```python
from build123d import *

# Parameters (mm, degrees)
SALIENTE_EXTRUIR1_DEPTH = 100
CORTAR_EXTRUIR2_DEPTH   = 101
CROQUIS4_R              = 5
CORTAR_EXTRUIR3_DEPTH   = 5
CROQUIS5_R              = 2.5
CORTAR_EXTRUIR4_DEPTH   = 55
CROQUIS6_R              = 5
CORTAR_EXTRUIR5_DEPTH   = 5
CROQUIS7_R              = 2.75
CORTAR_EXTRUIR6_DEPTH   = 55
CROQUIS8_R              = 2.75
CORTAR_EXTRUIR7_DEPTH   = 15
CROQUIS9_W              = 7.5
CROQUIS9_H              = 5
CORTAR_EXTRUIR8_DEPTH   = 12
CROQUIS10_W             = 7.5
CROQUIS10_H             = 5
CORTAR_EXTRUIR9_DEPTH   = 12
SALIENTE_EXTRUIR2_DEPTH = 10
SALIENTE_EXTRUIR3_DEPTH = 20
CORTAR_EXTRUIR10_DEPTH  = 10


with BuildPart() as part:
    # Croquis1 → Saliente-Extruir1 (new body)
    with BuildSketch(Plane.XY):
        with BuildLine():
            Line((-25.854679659, -27.188557242), (-25.854679659, -43))
            Line((-25.854679659, -43), (25.854679659, -43))
            Line((25.854679659, -43), (25.854679659, -27.188557242))
            Line((25.854679659, -27.188557242), (36.348456911, -13.489727661))
            ThreePointArc((36.348456911, -13.489727661), (27.329058454, -9.545941546), (23.385272339, -0.526543089))
            Line((23.385272339, -0.526543089), (10, -18))
            Line((10, -18), (-10, -18))
            Line((-10, -18), (-23.385272339, -0.526543089))
            ThreePointArc((-23.385272339, -0.526543089), (-27.329058454, -9.545941546), (-36.348456911, -13.489727661))
            Line((-36.348456911, -13.489727661), (-25.854679659, -27.188557242))
        make_face()
    extrude(amount=SALIENTE_EXTRUIR1_DEPTH)

    # Croquis3 → Cortar-Extruir2 (cut, through all)
    with BuildSketch(Plane.XY.offset(100)):
        Polygon((0, -33), (-29.159434589, -55.337135416), (29.159434589, -55.337135416), align=None)
    extrude(amount=-CORTAR_EXTRUIR2_DEPTH, mode=Mode.SUBTRACT)

    # Croquis4 → Cortar-Extruir3 (cut)
    with BuildSketch(Plane(origin=(15.930802982, -20.796453926, 0), x_dir=(-0.793848583, -0.608115471, 0), z_dir=(0.608115471, -0.793848583, 0))):
        with Locations((28.28993322, -85)):
            Circle(CROQUIS4_R)
        with Locations((28.28993322, -15)):
            Circle(CROQUIS4_R)
    extrude(amount=-CORTAR_EXTRUIR3_DEPTH, mode=Mode.SUBTRACT)

    # Croquis5 → Cortar-Extruir4 (cut)
    with BuildSketch(Plane(origin=(12.890225626, -16.827211008, 0), x_dir=(-0.793848583, -0.608115471, 0), z_dir=(0.608115471, -0.793848583, 0))):
        with Locations((28.28993322, -85)):
            Circle(CROQUIS5_R)
        with Locations((28.28993322, -15)):
            Circle(CROQUIS5_R)
    extrude(amount=-CORTAR_EXTRUIR4_DEPTH, mode=Mode.SUBTRACT)

    # Croquis6 → Cortar-Extruir5 (cut)
    with BuildSketch(Plane(origin=(-15.930802982, -20.796453926, 0), x_dir=(0.793848583, -0.608115471, 0), z_dir=(-0.608115471, -0.793848583, 0))):
        with Locations((28.28993322, 85)):
            Circle(CROQUIS6_R)
        with Locations((28.28993322, 15)):
            Circle(CROQUIS6_R)
    extrude(amount=-CORTAR_EXTRUIR5_DEPTH, mode=Mode.SUBTRACT)

    # Croquis7 → Cortar-Extruir6 (cut)
    with BuildSketch(Plane(origin=(-12.890225626, -16.827211008, 0), x_dir=(0.793848583, -0.608115471, 0), z_dir=(-0.608115471, -0.793848583, 0))):
        with Locations((28.28993322, 85)):
            Circle(CROQUIS7_R)
        with Locations((28.28993322, 15)):
            Circle(CROQUIS7_R)
    extrude(amount=-CORTAR_EXTRUIR6_DEPTH, mode=Mode.SUBTRACT)

    # Croquis8 → Cortar-Extruir7 (cut)
    with BuildSketch(Plane.XZ.offset(43)):
        with Locations((-20, 90)):
            Circle(CROQUIS8_R)
        with Locations((20, 90)):
            Circle(CROQUIS8_R)
        with Locations((20, 70)):
            Circle(CROQUIS8_R)
        with Locations((-20, 70)):
            Circle(CROQUIS8_R)
        with Locations((20, 50)):
            Circle(CROQUIS8_R)
        with Locations((-20, 50)):
            Circle(CROQUIS8_R)
        with Locations((20, 30)):
            Circle(CROQUIS8_R)
        with Locations((-20, 30)):
            Circle(CROQUIS8_R)
        with Locations((20, 10)):
            Circle(CROQUIS8_R)
        with Locations((-20, 10)):
            Circle(CROQUIS8_R)
    extrude(amount=-CORTAR_EXTRUIR7_DEPTH, mode=Mode.SUBTRACT)

    # Croquis9 → Cortar-Extruir8 (cut)
    with BuildSketch(Plane(origin=(25.854679659, 0, 0), x_dir=(0, 0, -1), z_dir=(1, 0, 0))):
        with Locations((-90, -35.094278621)):
            Rectangle(CROQUIS9_W, CROQUIS9_H)
        with Locations((-70, -35.094278621)):
            Rectangle(CROQUIS9_W, CROQUIS9_H)
        with Locations((-50, -35.094278621)):
            Rectangle(CROQUIS9_W, CROQUIS9_H)
        with Locations((-30, -35.094278621)):
            Rectangle(CROQUIS9_W, CROQUIS9_H)
        with Locations((-10, -35.094278621)):
            Rectangle(CROQUIS9_W, CROQUIS9_H)
    extrude(amount=-CORTAR_EXTRUIR8_DEPTH, mode=Mode.SUBTRACT)

    # Croquis10 → Cortar-Extruir9 (cut)
    with BuildSketch(Plane.ZY.offset(25.854679659)):
        with Locations((90, -35.094278621)):
            Rectangle(CROQUIS10_W, CROQUIS10_H)
        with Locations((70, -35.094278621)):
            Rectangle(CROQUIS10_W, CROQUIS10_H)
        with Locations((50, -35.094278621)):
            Rectangle(CROQUIS10_W, CROQUIS10_H)
        with Locations((30, -35.094278621)):
            Rectangle(CROQUIS10_W, CROQUIS10_H)
        with Locations((10, -35.094278621)):
            Rectangle(CROQUIS10_W, CROQUIS10_H)
    extrude(amount=-CORTAR_EXTRUIR9_DEPTH, mode=Mode.SUBTRACT)

    # Croquis11 → Saliente-Extruir2 (add)
    with BuildSketch(Plane(origin=(0, 0, 0), x_dir=(-1, 0, 0), z_dir=(0, 0, -1))):
        with BuildLine():
            Line((-50.332788561, 1.06673664), (-57.946904644, -27.188557242))
            Line((-57.946904644, -27.188557242), (-25.854679659, -27.188557242))
            Line((-25.854679659, -27.188557242), (-36.348456911, -13.489727661))
            ThreePointArc((-36.348456911, -13.489727661), (-46.610344914, -9.35270332), (-50.332788561, 1.06673664))
        make_face()
    extrude(amount=-SALIENTE_EXTRUIR2_DEPTH)

    # Croquis12 → Saliente-Extruir3 (add)
    with BuildSketch(Plane.XY.offset(10)):
        with BuildLine():
            Line((54.026124626, -27.188557242), (48.533618564, -6.806365636))
            ThreePointArc((48.533618564, -6.806365636), (50.035733702, -3.007505349), (50.332788561, 1.06673664))
            Line((50.332788561, 1.06673664), (57.946904644, -27.188557242))
            Line((57.946904644, -27.188557242), (54.026124626, -27.188557242))
        make_face()
    extrude(amount=SALIENTE_EXTRUIR3_DEPTH)

    # Croquis13 → Cortar-Extruir10 (cut)
    with BuildSketch(Plane(origin=(47.193210715, 12.717425139, 0), x_dir=(0, 0, -1), z_dir=(0.965556357, 0.260194009, 0))):
        with BuildLine():
            Line((-26.5, -35.129521687), (-21.5, -35.129521687))
            ThreePointArc((-21.5, -35.129521687), (-20.3, -36.329521687), (-21.5, -37.529521687))
            Line((-21.5, -37.529521687), (-26.5, -37.529521687))
            ThreePointArc((-26.5, -37.529521687), (-27.7, -36.329521687), (-26.5, -35.129521687))
        make_face()
        with BuildLine():
            Line((-26.5, -25.129521687), (-21.5, -25.129521687))
            ThreePointArc((-21.5, -25.129521687), (-20.3, -26.329521687), (-21.5, -27.529521687))
            Line((-21.5, -27.529521687), (-26.5, -27.529521687))
            ThreePointArc((-26.5, -27.529521687), (-27.7, -26.329521687), (-26.5, -25.129521687))
        make_face()
    extrude(amount=-CORTAR_EXTRUIR10_DEPTH, mode=Mode.SUBTRACT)


solid = part.part
```
Here's how the part is built. I have some questions about the finished solid (model axes, mm). A direction names the side the tool comes from. Round coordinates to 2 decimals unless told otherwise and drop trailing zeros. Order: outer loops, then holes, each group sorted by start corner. A loop starts at its lowest first (then second) coordinate and runs counter-clockwise, first axis right, second up. Notation, with made-up numbers: M 14.5,26 L 29.5,26 A17 ccw 29.5,48 Z; hole C 74,-23.75 d6. An arc over 180 degrees is marked long. Use CSV: the item, a comma, the result in double quotes.
1) I want a section at A-A (z = 70). Count the separate pieces of the cut face and the enclosed holes in it, then the cut area to 3 significant figures.
Taken from the geometry:
separate pieces,"3"
enclosed holes,"0"
area,"1,410 mm^2"
2) I need wall thicknesses on line 1 along Z through (x, y) = (-20, -39); line 2 along X through (y, z) = (-32.5, 18); line 3 along Z through (x, y) = (17, -28.5). Which ranges of each line are inside material? Lowest first, please. Write a range as [from, to].
Taken from the geometry:
line 1,"[0, 7.25], [12.75, 27.25], [32.75, 47.25], [52.75, 67.25], [72.75, 87.25], [92.75, 100]"
line 2,"[-25.85, -7.57], [-5.7, 5.7], [7.57, 25.85]"
line 3,"[0, 13.94], [16.06, 83.94], [86.06, 100]"
3) On a 3-axis mill with a long thin cutter (end or side, diameter ignored), from which of +Z, -Z, +X, -X, +Y, -Y can I reach the whole of each face in a straight line? I mean faces 1 (the flat face through (-13.855, -35, 50)), 2 (the flat face through (54.53, -21.69, 24.04)), 3 (the flat face through (-6.436, -37.93, 50.7)), 4 (the flat face through (55.156, -24.005, 23.965)). Say none if no direction works.
Taken from the geometry:
face 1,"-X"
face 2,"+X"
face 3,"+Z, -Z, -Y"
face 4,"none"
4) I want a section at D-D (x = 45). List the corners of the cut face in (y, z) for me.
Taken from the geometry:
outline,"M -27.19,0 L -10.78,0 L -10.78,10 L -27.19,10 Z"
5) I'm going to push flat-ended pins straight in: P1, Ø9, axis at x = 20, z = 10, coming from the -Y side; P2, Ø4, axis at y = -36, z = 9, coming from the +X side; P3, Ø17.5, axis at y = -34.5, z = 29.5, coming from the -X side; P4, Ø5, axis at x = -25.5, z = 44.5, coming from the +Y side. Where does each tip first touch, or does it pass through?
Taken from the geometry:
P1,"y = -43"
P2,"x = 25.85"
P3,"x = -26.96"
P4,"y = -0.53"
6) If we mould it in two halves opening along Y, with no side actions, what happens to faces 5 (the flat face through (20, -28, 30)), 6 (the flat face through (-25.855, -38, 49)), 7 (the flat face through (-17, -32.594, 49))? For each: pulls with the +Y half, pulls with the -Y half, needs draft (parallel to the pull), parting line crosses it, or undercut.
Taken from the geometry:
face 5,"pulls with the -Y half"
face 6,"needs draft"
face 7,"undercut"
